```python
from build123d import *

# Parameters (mm, degrees)
SKETCH_W     = 6.6
SKETCH_H     = 15
PAD_DEPTH    = 1
SKETCH001_W  = 2.925
SKETCH001_H  = 2
PAD001_DEPTH = 1
PAD002_DEPTH = 6.6
SKETCH003_W  = 0.75
SKETCH003_H  = 3
POCKET_DEPTH = 15.001


with BuildPart() as part:
    # Sketch → Pad (new body)
    with BuildSketch(Plane.XY):
        with Locations((0, 7.5)):
            Rectangle(SKETCH_W, SKETCH_H)
    extrude(amount=PAD_DEPTH)

    # Sketch001 → Pad001 (new body)
    with BuildSketch(Plane.XY.offset(1)):
        with Locations((-1.8375, 1)):
            Rectangle(SKETCH001_W, SKETCH001_H)
        with Locations((1.8375, 1)):
            Rectangle(SKETCH001_W, SKETCH001_H)
    extrude(amount=PAD001_DEPTH)

    # Sketch002 → Pad002 (new body)
    with BuildSketch(Plane(origin=(-3.3, 0, 0), x_dir=(0, -1, 0), z_dir=(-1, 0, 0))):
        Polygon((-15, 0), (-12.25, 0), (-12.25, 4), (-13.25, 4), (-13.25, 3), (-14, 3), (-14, 4), (-15, 4), align=None)
    extrude(amount=-PAD002_DEPTH)

    # Sketch003 → Pocket (cut, through all)
    with BuildSketch(Plane.XZ):
        with Locations((0, 2.5)):
            Rectangle(SKETCH003_W, SKETCH003_H)
    extrude(amount=-POCKET_DEPTH, mode=Mode.SUBTRACT)


solid = part.part
```
Source: CAD feature listing. Evaluate the final solid. Frame: model axes, mm. A direction names the side the tool comes from. Give positions to 0.01 mm unless a question says otherwise; leave off trailing zeros. Loops run counter-clockwise (first coordinate to the right, second up) from the corner with the lowest first, then second, coordinate; pieces in that order, holes last. Notation, with made-up numbers: (7, 79.5) -> (27, 79.5) arc R24 ccw to (27, 118.5) -> close; hole circle Ø10 at (20, 51). An arc over 180 degrees is marked (long way). Put each result on its own line as item: value. Start each with the question number.
1) Material intervals for probe 1 along Y at (x, z) = (-2.5, 1.7); probe 2 along Y at (x, z) = (1.5, 3.55); probe 3 along X at (y, z) = (1.25, 1.15) (3 decimals), sorted ascending.
2) Reachability of faces 1 (the face through (-2, 1, 2)), 2 (the face through (1.8, 14.5, 4)), 3 (the face through (1.8, 13.25, 3.5)), 4 (the face through (-0.375, 1, 1.5)) from +Z, -Z, +X, -X, +Y, -Y: full face, straight path, thin tool, end or side. Return the list, or none.
3) Contact query for flat-ended pins moving along their axis: P1, Ø2, axis at x = -2, y = 1, coming from the +Z side; P2, Ø1.5, axis at x = -2, y = 7.5, coming from the +Z side; P3, Ø1.1, axis at x = -2, z = 3.5, coming from the -Y side. Output: stop coordinate, or through.
4) Cut plane B-B (y = 12.75). Return loops of the section in (x, z) (3 decimals).
5) Cut plane D-D (z = 3.35). Return loops of the section in (x, y) (3 decimals), then the cut area to 3 significant figures.
6) Cut plane C-C (x = 2.5). Return loops of the section in (y, z), then the cut area to 3 significant figures.
7) Draft query along X for faces 5 (the face through (-1.9, 14, 3.5)), 6 (the face through (-3.3, 9.1, 0.6)), 7 (the face through (-0.375, 14, 2)), 8 (the face through (0.375, 1, 1.5)). Return one class per face: released by +X, released by -X, zero draft, split by the parting line, or undercut.
8) Cut plane A-A (z = 1.2). Return loops of the section in (x, y) (3 decimals), then the cut area to 3 significant figures.
Results are:
1. probe 1: y = 0 to 2, 12.25 to 15
1. probe 2: y = 12.25 to 13.25, 14 to 15
1. probe 3: x = -3.3 to -0.375, 0.375 to 3.3
2. face 1: +Z, +X, -X, -Y
2. face 2: +Z, +X, -X, +Y, -Y
2. face 3: +Z, +X, -X
2. face 4: +Z, +Y, -Y
3. P1: stops at z = 2
3. P2: stops at z = 1
3. P3: stops at y = 12.25
4. outline: (-3.3, 0) -> (3.3, 0) -> (3.3, 4) -> (0.375, 4) -> (0.375, 1) -> (-0.375, 1) -> (-0.375, 4) -> (-3.3, 4) -> close
5. outline: (-3.3, 12.25) -> (-0.375, 12.25) -> (-0.375, 13.25) -> (-3.3, 13.25) -> close; (-3.3, 14) -> (-0.375, 14) -> (-0.375, 15) -> (-3.3, 15) -> close; (0.375, 12.25) -> (3.3, 12.25) -> (3.3, 13.25) -> (0.375, 13.25) -> close; (0.375, 14) -> (3.3, 14) -> (3.3, 15) -> (0.375, 15) -> close
5. area: 11.7 mm2
6. outline: (0, 0) -> (15, 0) -> (15, 4) -> (14, 4) -> (14, 3) -> (13.25, 3) -> (13.25, 4) -> (12.25, 4) -> (12.25, 1) -> (2, 1) -> (2, 2) -> (0, 2) -> close
6. area: 24.5 mm2
7. face 5: zero draft
7. face 6: released by -X
7. face 7: undercut
7. face 8: undercut
8. outline: (-3.3, 0) -> (-0.375, 0) -> (-0.375, 2) -> (-3.3, 2) -> close; (-3.3, 12.25) -> (-0.375, 12.25) -> (-0.375, 15) -> (-3.3, 15) -> close; (0.375, 0) -> (3.3, 0) -> (3.3, 2) -> (0.375, 2) -> close; (0.375, 12.25) -> (3.3, 12.25) -> (3.3, 15) -> (0.375, 15) -> close
8. area: 27.8 mm2
